Input: dimensioned drawing with shaded views. Units: mm. Origin: part minimum x, y, z. Round coordinates to 2 decimals unless told otherwise and drop trailing zeros. Loops run counter-clockwise (first coordinate to the right, second up) from the corner with the lowest first, then second, coordinate; pieces in that order, holes last. Notation, with made-up numbers: (44, 67) -> (68, 67) arc R24 ccw to (68, 91) -> close; hole circle Ø6 at (44.25, 67). An arc over 180 degrees is marked (long way). Answer as a JSON object with one key per item and string values.
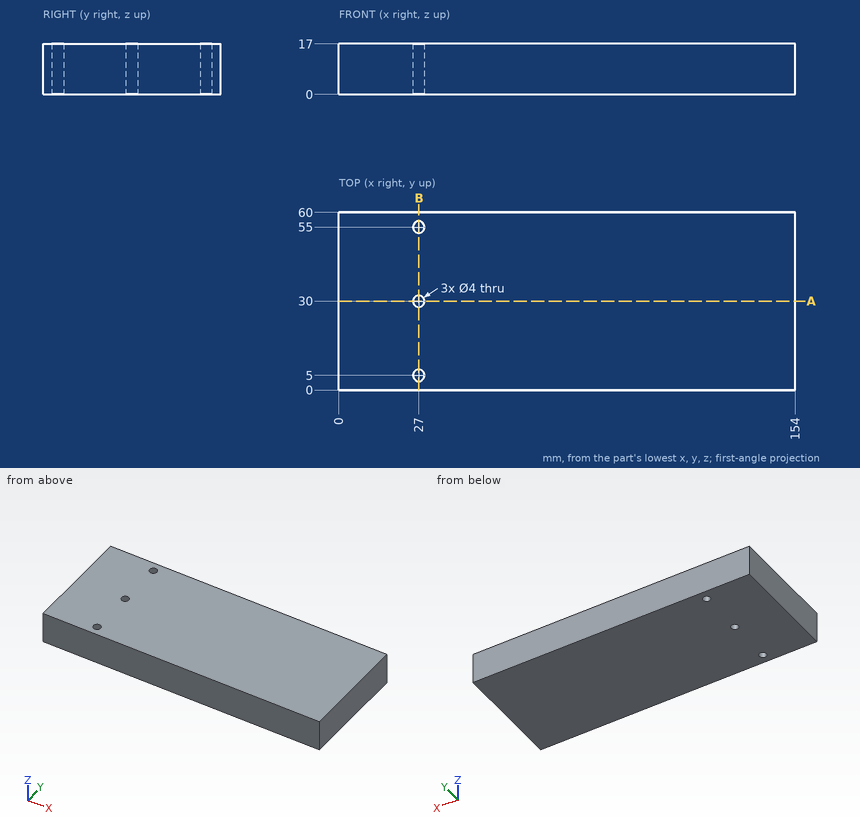
1) Ray query, probe 1 along Y at (x, z) = (27, 10.5); probe 2 along X at (y, z) = (31, 11.5); probe 3 along X at (y, z) = (54.5, 12.5). Return the intervals inside material, ascending.
Output:
{"probe 1": "y = 0 to 3, 7 to 28, 32 to 53, 57 to 60", "probe 2": "x = 0 to 25.27, 28.73 to 154", "probe 3": "x = 0 to 25.06, 28.94 to 154"}
2) Contact query for a flat-ended pin moving along its axis: P1, Ø6, axis at y = 15.5, z = 2, coming from the -X side. Output: stop coordinate, or through.
Output:
{"P1": "stops at x = 0"}
3) Section A-A, the plane y = 30. Output: boundary loops of the cut face in (x, z), plus the area to 3 significant figures.
Output:
{"outline": "(0, 0) -> (25, 0) -> (25, 17) -> (0, 17) -> close; (29, 0) -> (154, 0) -> (154, 17) -> (29, 17) -> close", "area": "2,550 mm^2"}
4) Section B-B, the plane x = 27. Output: boundary loops of the cut face in (y, z), plus the area to 3 significant figures.
Output:
{"outline": "(0, 0) -> (3, 0) -> (3, 17) -> (0, 17) -> close; (7, 0) -> (28, 0) -> (28, 17) -> (7, 17) -> close; (32, 0) -> (53, 0) -> (53, 17) -> (32, 17) -> close; (57, 0) -> (60, 0) -> (60, 17) -> (57, 17) -> close", "area": "816 mm^2"}
